Geometry check sheet. Reference: the model listing, model coordinates, mm. A direction names the side the tool comes from. Give positions to 0.01 mm unless a question says otherwise; leave off trailing zeros. Order: outer loops, then holes, each group sorted by start corner. A loop starts at its lowest first (then second) coordinate and runs counter-clockwise, first axis right, second up. Notation, with made-up numbers: M 5,77.25 L 29,77.25 A34 cw 29,111.25 Z; hole C -11,80 d11. An arc over 180 degrees is marked long. One line per question, with ' | ' between items. Start each with the question number.
from build123d import *

# Parameters (mm, degrees)
SKETCH1_W           = 24
SKETCH1_H           = 13
BOSS_EXTRUDE1_DEPTH = 15
CUT_EXTRUDE1_DEPTH  = 13
SKETCH3_R           = 2.6
CUT_EXTRUDE2_DEPTH  = 2
CUT_EXTRUDE3_DEPTH  = 13
BOSS_EXTRUDE3_DEPTH = 8
SKETCH6_R           = 1.6
BOSS_EXTRUDE4_DEPTH = 3
FILLET1_R           = 2
CUT_EXTRUDE8_DEPTH  = 28.009257672
CUT_EXTRUDE9_DEPTH  = 12


with BuildPart() as part:
    # Sketch1 → Boss-Extrude1 (new body)
    with BuildSketch(Plane(origin=(0, 0, 0), x_dir=(1, 0, 0), z_dir=(0, 1, 0))):
        Polygon((-12, -6.5), (-12, 6.5), (-17, 0), align=None)
        Rectangle(SKETCH1_W, SKETCH1_H)
        Polygon((17, 0), (12, -6.5), (12, 6.5), align=None)
    extrude(amount=BOSS_EXTRUDE1_DEPTH)

    # Sketch2 → Cut-Extrude1 (cut)
    with BuildSketch(Plane.XZ):
        Polygon((-11.015197005, 4.5), (-14.476735467, 0), (-11.015197005, -4.5), (0, -4.5), (0, 4.5), align=None)
        Polygon((0, 4.5), (0, -4.5), (11.015197005, -4.5), (14.476735467, 0), (11.015197005, 4.5), align=None)
    extrude(amount=-CUT_EXTRUDE1_DEPTH, mode=Mode.SUBTRACT)

    # Sketch3 → Cut-Extrude2 (cut)
    with BuildSketch(Plane(origin=(0, 15, 0), x_dir=(1, 0, 0), z_dir=(0, 1, 0))):
        with Locations(Location((-9.5, 0, 0), (0, 0, 270))):
            Circle(SKETCH3_R)
        with Locations(Location((9.5, 0, 0), (0, 0, 270))):
            Circle(SKETCH3_R)
    extrude(amount=-CUT_EXTRUDE2_DEPTH, mode=Mode.SUBTRACT)

    # Sketch4 → Cut-Extrude3 (cut)
    with BuildSketch(Plane.XZ.offset(-13)):
        Polygon((-6.4, 2.5), (-5.5, 2.5), (-5.5, 4), (-13.5, 4), (-13.5, -4), (-5.5, -4), (-5.5, -2.5), (-6.4, -2.5), (-6.4, -3.1), (-12.092120082, -3.1), (-12.6, -2.439756107), (-12.6, 2.439756107), (-12.082269007, 3.1), (-6.4, 3.1), align=None)
        Polygon((6.4, 2.5), (6.4, 3.1), (12.082269007, 3.1), (12.6, 2.439756107), (12.6, -2.439756107), (12.092120082, -3.1), (6.4, -3.1), (6.4, -2.5), (5.5, -2.5), (5.5, -4), (13.5, -4), (13.5, 4), (5.5, 4), (5.5, 2.5), align=None)
    extrude(amount=CUT_EXTRUDE3_DEPTH, mode=Mode.SUBTRACT)

    # Sketch5 → Boss-Extrude3 (add)
    with BuildSketch(Plane.XZ.offset(-13)):
        Polygon((-6.4, -3.1), (-12.6, -3.1), (-12.6, 3.1), (-6.4, 3.1), (-6.4, 2.5), (-5.5, 2.5), (-5.5, 4), (-13.5, 4), (-13.5, -4), (-5.5, -4), (-5.5, -2.5), (-6.4, -2.5), align=None)
        Polygon((12.6, -3.1), (12.6, 3.1), (6.4, 3.1), (6.4, 2.5), (5.5, 2.5), (5.5, 4), (13.5, 4), (13.5, -4), (5.5, -4), (5.5, -2.5), (6.4, -2.5), (6.4, -3.1), align=None)
    extrude(amount=BOSS_EXTRUDE3_DEPTH)

    # Sketch6 → Boss-Extrude4 (add)
    # profile 1 of 2: a face of its own
    with BuildSketch(Plane(origin=(0, 0, 0), x_dir=(1, 0, 0), z_dir=(0, 1, 0))):
        Polygon((21.5, 3.25), (14.5, 3.25), (17, 0), (14.5, -3.25), (21.5, -3.25), align=None)
        with Locations(Location((19.25, 0, 0), (0, 0, 270))):
            Circle(SKETCH6_R, mode=Mode.SUBTRACT)
    # profile 2 of 2: a face of its own
    with BuildSketch(Plane(origin=(0, 0, 0), x_dir=(1, 0, 0), z_dir=(0, 1, 0))):
        Polygon((-17, 0), (-14.5, 3.25), (-21.5, 3.25), (-21.5, -3.25), (-14.5, -3.25), align=None)
        with Locations(Location((-19.25, 0, 0), (0, 0, 270))):
            Circle(SKETCH6_R, mode=Mode.SUBTRACT)
    extrude(amount=BOSS_EXTRUDE4_DEPTH)

    # Fillet1
    fillet1_edges = [part.edges().sort_by_distance(p)[0] for p in [
        (-17, 9, 0),
        (-12, 7.5, -6.5),
        (12, 7.5, -6.5),
        (17, 9, 0),
        (12, 7.5, 6.5),
        (-12, 7.5, 6.5),
    ]]
    fillet(fillet1_edges, radius=FILLET1_R)

    # Sketch8 → Cut-Extrude8 (cut, through all)
    with BuildSketch(Plane.XZ):
        with BuildLine():
            Line((-14.5, -3.25), (-21.5, -3.25))
            Line((-21.5, -3.25), (-21.5, 3.25))
            Line((-21.5, 3.25), (-14.5, 3.25))
            Line((-14.5, 3.25), (-12.600444983, 5.719421522))
            ThreePointArc((-12.600444983, 5.719421522), (-11.89870053, 6.294274651), (-11.015197005, 6.5))
            Line((-11.015197005, 6.5), (11.015197005, 6.5))
            ThreePointArc((11.015197005, 6.5), (11.89870053, 6.294274651), (12.600444983, 5.719421522))
            Line((12.600444983, 5.719421522), (14.5, 3.25))
            Line((14.5, 3.25), (21.5, 3.25))
            Line((21.5, 3.25), (21.5, -3.25))
            Line((21.5, -3.25), (14.5, -3.25))
            Line((14.5, -3.25), (12.600444983, -5.719421522))
            ThreePointArc((12.600444983, -5.719421522), (11.89870053, -6.294274651), (11.015197005, -6.5))
            Line((11.015197005, -6.5), (-11.015197005, -6.5))
            ThreePointArc((-11.015197005, -6.5), (-11.89870053, -6.294274651), (-12.600444983, -5.719421522))
            Line((-12.600444983, -5.719421522), (-14.5, -3.25))
        make_face()
        with BuildLine():
            Line((-14.45075985, -3.15), (-21.4, -3.15))
            Line((-21.4, -3.15), (-21.4, 3.15))
            Line((-21.4, 3.15), (-14.45075985, 3.15))
            Line((-14.45075985, 3.15), (-12.521182584, 5.658450446))
            ThreePointArc((-12.521182584, 5.658450446), (-11.854525354, 6.204560918), (-11.015197005, 6.4))
            Line((-11.015197005, 6.4), (11.015197005, 6.4))
            ThreePointArc((11.015197005, 6.4), (11.854525354, 6.204560918), (12.521182584, 5.658450446))
            Line((12.521182584, 5.658450446), (14.45075985, 3.15))
            Line((14.45075985, 3.15), (21.4, 3.15))
            Line((21.4, 3.15), (21.4, -3.15))
            Line((21.4, -3.15), (14.45075985, -3.15))
            Line((14.45075985, -3.15), (12.521182584, -5.658450446))
            ThreePointArc((12.521182584, -5.658450446), (11.854525354, -6.204560918), (11.015197005, -6.4))
            Line((11.015197005, -6.4), (-11.015197005, -6.4))
            ThreePointArc((-11.015197005, -6.4), (-11.854525354, -6.204560918), (-12.521182584, -5.658450446))
            Line((-12.521182584, -5.658450446), (-14.45075985, -3.15))
        make_face(mode=Mode.SUBTRACT)
    extrude(amount=-CUT_EXTRUDE8_DEPTH, mode=Mode.SUBTRACT)

    # Sketch9 → Cut-Extrude9 (cut)
    with BuildSketch(Plane(origin=(0, 15, 0), x_dir=(1, 0, 0), z_dir=(0, 1, 0))):
        with BuildLine():
            Line((14.576923077, -3.15), (14.45075985, -3.15))
            Line((14.45075985, -3.15), (14.527682927, -3.05))
            Line((14.527682927, -3.05), (15.982721046, -1.158450446))
            ThreePointArc((15.982721046, -1.158450446), (16.376735467, 0), (15.982721046, 1.158450446))
            Line((15.982721046, 1.158450446), (14.527682927, 3.05))
            Line((14.527682927, 3.05), (14.45075985, 3.15))
            Line((14.45075985, 3.15), (14.576923077, 3.15))
            Line((14.576923077, 3.15), (16.061983445, 1.219421522))
            ThreePointArc((16.061983445, 1.219421522), (16.476735467, 0), (16.061983445, -1.219421522))
            Line((16.061983445, -1.219421522), (14.576923077, -3.15))
        make_face()
        with BuildLine():
            Line((-14.45075985, -3.15), (-14.576923077, -3.15))
            Line((-14.576923077, -3.15), (-16.061983445, -1.219421522))
            ThreePointArc((-16.061983445, -1.219421522), (-16.476735467, 0), (-16.061983445, 1.219421522))
            Line((-16.061983445, 1.219421522), (-14.576923077, 3.15))
            Line((-14.576923077, 3.15), (-14.45075985, 3.15))
            Line((-14.45075985, 3.15), (-14.527682927, 3.05))
            Line((-14.527682927, 3.05), (-15.982721046, 1.158450446))
            ThreePointArc((-15.982721046, 1.158450446), (-16.376735467, 0), (-15.982721046, -1.158450446))
            Line((-15.982721046, -1.158450446), (-14.527682927, -3.05))
            Line((-14.527682927, -3.05), (-14.45075985, -3.15))
        make_face()
    extrude(amount=-CUT_EXTRUDE9_DEPTH, mode=Mode.SUBTRACT)


solid = part.part
Item 1: Cross-section at D-D, the plane z = -5.25. Record the cut outline in (x, y).
Item 2: Mould release check, pull along X, two halves, no side actions. Record for faces 1 (the flat face through (-21.4, 1, 0)), 2 (the flat face through (-10, 9, 3.1)), 3 (the flat face through (17, 3, 0)): released by +X, released by -X, zero draft, split by the parting line, or undercut.
Item 3: Material ranges on line 1 along X through (y, z) = (9.75, 1); line 2 along X through (y, z) = (8.75, 0.25); line 3 along X through (y, z) = (11.5, 1.75), recorded low to high.
Item 4: Set-up check for faces 4 (the cylindrical face through (-17.664, 1.479, -0.208)), 5 (the flat face through (12, 3, 4)): record each of +Z, -Z, +X, -X, +Y, -Y from which the full face is reachable in a straight line by a thin tool's end or side.
Item 5: Cross-section at A-A, the plane x = -19.25. Record the cut outline in (y, z), plus the area to 3 significant figures.
Item 6: Depth check by flat-ended pin: pin 1 (0.8 mm diameter, centred on y = 8, z = -3.5, fed in from -X); pin 2 (0.6 mm diameter, centred on x = -12.5, y = 1.5, fed in from -Z); pin 3 (4 mm diameter, centred on x = -10, z = 1, fed in from -Y). Enter the tip coordinate at first touch or a pass-through.
Item 7: Cross-section at C-C, the plane y = 8.5. State how many separate pieces and enclosed holes the cut face has, plus the area to 3 significant figures.
Item 8: Cross-section at B-B, the plane x = -9.5. Record the cut outline in (y, z).
Outcome:
1) outline: M -12.84,0 L 12.84,0 L 12.84,15 L -12.84,15 Z
2) face 1: released by -X | face 2: undercut | face 3: zero draft
3) line 1: x = -16.09 to -13.71, -13.5 to -12.6, 12.6 to 13.5, 13.71 to 16.09 | line 2: x = -16.36 to -14.28, -13.5 to -12.6, 12.6 to 13.5, 14.28 to 16.36 | line 3: x = -15.53 to -12.6, 12.6 to 15.53
4) face 4: +Y, -Y | face 5: -Y
5) outline: M 0,-3.15 L 3,-3.15 L 3,-1.6 L 0,-1.6 Z; M 0,1.6 L 3,1.6 L 3,3.15 L 0,3.15 Z | area: 9.30 mm²
6) pin 1: stops at x = -14.49 | pin 2: stops at z = -5.99 | pin 3: stops at y = 13
7) separate pieces: 1 | enclosed holes: 3 | area: 169 mm²
8) outline: M 0,-6.4 L 15,-6.4 L 15,-2.6 L 13,-2.6 L 13,-3.1 L 5,-3.1 L 5,-4 L 13,-4 L 13,-4.5 L 0,-4.5 Z; M 0,4.5 L 13,4.5 L 13,4 L 5,4 L 5,3.1 L 13,3.1 L 13,2.6 L 15,2.6 L 15,6.4 L 0,6.4 Z
